Could you check a few things on this model? Use its own coordinates, in mm. A direction names the side the tool comes from. Give positions to 0.01 mm unless a question says otherwise; leave off trailing zeros. Order: outer loops, then holes, each group sorted by start corner. A loop starts at its lowest first (then second) coordinate and runs counter-clockwise, first axis right, second up. Notation, with made-up numbers: (-37.75, -1) -> (8.25, -1) arc R11 ccw to (8.25, 11) -> close; hole circle Ø4 at (-2, 54). An arc over 180 degrees is marked (long way). One line per item, written item: value.
```python
from build123d import *

# Parameters (mm, degrees)
F1_DEPTH       = 7.5
F2_R           = 1
F4_D           = 5.5
F4_CSINK_D     = 11.2
F4_CSINK_ANGLE = 90
F5_R           = 7.5


with BuildPart() as f1:
    # F0 (on Right) → F1 (new body, symmetric)
    with BuildSketch(Plane.YZ):
        Polygon((-67, 0), (-62, 0), (-62, 6), (-67, 3.917779892), align=None)
        Polygon((-62, 6), (-44.9935843937, 6), (-49.9935843937, 11), align=None)
        Polygon((-12, 0), (-12, 6), (-44.9935843937, 6), (-62, 6), (-62, 0), align=None)
        Polygon((-62, -6), (-62, 0), (-67, 0), (-67, -3.917779892), align=None)
        Polygon((-49.9935843937, -11), (-44.9935843937, -6), (-62, -6), align=None)
        Polygon((-12, -6), (-12, 0), (-62, 0), (-62, -6), (-44.9935843937, -6), align=None)
        Polygon((0, 0), (0, 30), (-12, 30), (-12, 6), (-12, 0), align=None)
        Polygon((0, -30), (0, 0), (-12, 0), (-12, -6), (-12, -30), align=None)
    extrude(amount=F1_DEPTH, both=True)

    # F2
    f2_edges = [f1.edges().sort_by_distance(p)[0] for p in [
        (0, -49.993584, 11),
        (0, -67, 3.91778),
        (0, -67, -3.91778),
        (0, -49.993584, -11),
    ]]
    fillet(f2_edges, radius=F2_R)

    # F4 (through all)
    with Locations(Plane.XZ.offset(12)):
        with Locations((0, 20), (0, -20)):
            CounterSinkHole(F4_D / 2, F4_CSINK_D / 2, counter_sink_angle=F4_CSINK_ANGLE)

    # F5
    f5_edges = [f1.edges().sort_by_distance(p)[0] for p in [
        (0, -12, 6),
        (0, -12, -6),
    ]]
    fillet(f5_edges, radius=F5_R)


solid = f1.part
```
1) Suppose I cut it at A-A, the plane x = 0. State how many separate pieces and enclosed holes the cut face has, then the cut area to 3 significant figures.
Answer below:
separate pieces: 3
enclosed holes: 0
area: 1,330 mm2
2) For faces 1 (the flat face through (0, -6, -30)), 2 (the flat face through (2, -12, 26)), 3 (the flat face through (3, -12, -25)), 4 (the cylindrical face through (0.105, -14.139, -8.255)), 5 (the flat face through (0, -32, 6)), which set-ups out of +Z, -Z, +X, -X, +Y, -Y let a thin tool reach every point of the face, with its end or its side?
Answer below:
face 1: -Z, +X, -X, +Y, -Y
face 2: +Z, +X, -X, -Y
face 3: -Z, +X, -X, -Y
face 4: -Z, +X, -X
face 5: +Z, +X, -X
3) Suppose I cut it at D-D, the plane y = -52. Write out the boundary of the cut face in (x, z), then the cut area to 3 significant figures.
Answer below:
outline: (-7.5, -10.16) -> (7.5, -10.16) -> (7.5, 10.16) -> (-7.5, 10.16) -> close
area: 305 mm2
4) Suppose I cut it at C-C, the plane y = -36. Write out the boundary of the cut face in (x, z), then the cut area to 3 significant figures.
Answer below:
outline: (-7.5, -6) -> (7.5, -6) -> (7.5, 6) -> (-7.5, 6) -> close
area: 180 mm2
5) For P1, Ø5, axis at x = 0, z = -20, coming from the -Y side; P2, Ø3, axis at x = 3, z = 18, coming from the -Y side; P3, Ø4.5, axis at x = -2.5, z = 23.5, coming from the -Y side; P4, Ø4.5, axis at x = -2, y = -35, coming from the +Z side, each with a flat end and sliding along its axis, tell me the tip position at first contact or that it passes through.
Answer below:
P1: passes through
P2: stops at y = -11.51
P3: stops at y = -12
P4: stops at z = 6
6) If I drill on line 1 along Z through (x, y) = (0, -4); line 2 along X through (y, z) = (-2.5, -20); line 3 along Z through (x, y) = (-6.5, -23), over which ranges is the centre line in solid material (lowest first)?
Answer below:
line 1: z = -30 to -22.75, -17.25 to 17.25, 22.75 to 30
line 2: x = -7.5 to -2.75, 2.75 to 7.5
line 3: z = -6 to 6
7) We'd pull the mould along Y, two halves only. Please class faces 6 (the conical face through (0.376, -9.288, -17.136)), 7 (the flat face through (0, 0, 0)), 8 (the flat face through (0, -32, -6)): +Y half, -Y half, draft (parallel to the pull), parting line (faces both ways), or undercut.
Answer below:
face 6: -Y half
face 7: +Y half
face 8: undercut
8) Suppose I cut it at B-B, the plane z = 20. Write out the boundary of the cut face in (x, y), then the cut area to 3 significant figures.
Answer below:
outline: (-7.5, -12) -> (-5.6, -12) -> (-2.75, -9.15) -> (-2.75, 0) -> (-7.5, 0) -> close; (2.75, -9.15) -> (5.6, -12) -> (7.5, -12) -> (7.5, 0) -> (2.75, 0) -> close
area: 106 mm2
